from build123d import *

# Parameters (mm, degrees)
SKETCH_2_W          = 15.8
SKETCH_2_H          = 7.8
EXTRUDE_1_DEPTH     = 9.6
SKETCH_3_R          = 2.609387956
EXTRUDE_2_DEPTH     = 1.7
SKETCH_4_R          = 1.6
CUT_EXTRUDE_1_DEPTH = 1.7
SKETCH_5_R          = 1.6
CUT_EXTRUDE_2_DEPTH = 1.7


with BuildPart() as part:
    # Эскиз2 → Бобышка-Вытянуть1 (new body)
    with BuildSketch(Plane(origin=(0, 0, 0), x_dir=(1, 0, 0), z_dir=(0, 1, 0))):
        Rectangle(SKETCH_2_W, SKETCH_2_H)
    extrude(amount=EXTRUDE_1_DEPTH)

    # Эскиз3 → Бобышка-Вытянуть2 (add)
    with BuildSketch(Plane(origin=(0, 9.6, 0), x_dir=(1, 0, 0), z_dir=(0, 1, 0))):
        with Locations(Location((4, 0, 0), (0, 0, 270))):
            Circle(SKETCH_3_R)
        with Locations(Location((-3.874, 0, 0), (0, 0, 270))):
            Circle(SKETCH_3_R)
    extrude(amount=EXTRUDE_2_DEPTH)

    # Эскиз4 → Вырез-Вытянуть1 (cut)
    with BuildSketch(Plane(origin=(0, 11.3, 0), x_dir=(1, 0, 0), z_dir=(0, 1, 0))):
        with Locations(Location((-3.874, 0, 0), (0, 0, 270))):
            Circle(SKETCH_4_R)
    extrude(amount=-CUT_EXTRUDE_1_DEPTH, mode=Mode.SUBTRACT)

    # Эскиз5 → Вырез-Вытянуть2 (cut)
    with BuildSketch(Plane(origin=(0, 11.3, 0), x_dir=(1, 0, 0), z_dir=(0, 1, 0))):
        with Locations(Location((4, 0, 0), (0, 0, 270))):
            Circle(SKETCH_5_R)
    extrude(amount=-CUT_EXTRUDE_2_DEPTH, mode=Mode.SUBTRACT)


solid = part.part
Part model, mm, in its own coordinate system. A direction names the side the tool comes from. Round coordinates to 2 decimals unless told otherwise and drop trailing zeros. Write each loop counter-clockwise with the first axis right and the second up, starting at its lowest first coordinate (ties: lowest second). Pieces come first, ordered by that corner, then holes. Notation, with made-up numbers: M 25,79 L 44,79 A16 cw 44,109 Z; hole C -4.75,-4 d7. An arc over 180 degrees is marked long. Return JSON: item names as keys, results as strings. Group by question number.
(1) Saw through at B-B on z = 0. Write the cut outline in (x, y), then the cut area to 3 significant figures.
(2) Saw through at D-D on x = -5. Write the cut outline in (y, z), then the cut area to 3 significant figures.
(3) Saw through at C-C on y = 10. Write the cut outline in (x, z), then the cut area to 3 significant figures.
(4) Pin check, flat tip, straight feed: pin 1 Ø1 at (x, z) = (-4.5, -1) entering from +Y. Stop position of the tip, or through.
(5) Drill centre lines: probe 1 along X at (y, z) = (10.35, 0); probe 2 along Y at (x, z) = (4.25, -3). Where is each one in solid material? Low to high.
(6) Which spindle directions (+Z, -Z, +X, -X, +Y, -Y) get a long thin tool onto all of the face, cutting with end or side? Do faces 1 (the face through (-4, 11.3, 2)), 2 (the face through (-1.287, 10.438, -0.34)). Say none if no direction does.
(7) Saw through at A-A on x = 4. Write the cut outline in (y, z).
(8) Two-plate mould, pull along Z, no slides. Class faces 3 (the face through (0, 5, 3.9)), 4 (the face through (4, 9.6, 0)), 5 (the face through (7.9, 5, 0)): +Z half, -Z half, draft (parallel to the pull), parting line (faces both ways), or undercut.
Returned:
{
 "1": {"outline": "M -7.9,0 L 7.9,0 L 7.9,9.6 L 6.61,9.6 L 6.61,11.3 L 5.6,11.3 L 5.6,9.6 L 2.4,9.6 L 2.4,11.3 L 1.39,11.3 L 1.39,9.6 L -1.26,9.6 L -1.26,11.3 L -2.27,11.3 L -2.27,9.6 L -5.47,9.6 L -5.47,11.3 L -6.48,11.3 L -6.48,9.6 L -7.9,9.6 Z", "area": "159 mm²"},
 "2": {"outline": "M 0,-3.9 L 9.6,-3.9 L 9.6,-2.35 L 11.3,-2.35 L 11.3,-1.14 L 9.6,-1.14 L 9.6,1.14 L 11.3,1.14 L 11.3,2.35 L 9.6,2.35 L 9.6,3.9 L 0,3.9 Z", "area": "79.0 mm²"},
 "3": {"outline": "C -3.87,0 d5.22; C 4,0 d5.22; hole C -3.87,0 d3.2; hole C 4,0 d3.2", "area": "26.7 mm²"},
 "4": {"pin 1": "y = 11.3"},
 "5": {"probe 1": "-6.48 to -5.47, -2.27 to -1.26, 1.39 to 2.4, 5.6 to 6.61", "probe 2": "0 to 9.6"},
 "6": {"face 1": "+Z, -Z, +X, -X, +Y", "face 2": "+Y"},
 "7": {"outline": "M 0,-3.9 L 9.6,-3.9 L 9.6,-2.61 L 11.3,-2.61 L 11.3,-1.6 L 9.6,-1.6 L 9.6,1.6 L 11.3,1.6 L 11.3,2.61 L 9.6,2.61 L 9.6,3.9 L 0,3.9 Z"},
 "8": {"face 3": "+Z half", "face 4": "undercut", "face 5": "draft"}
}
